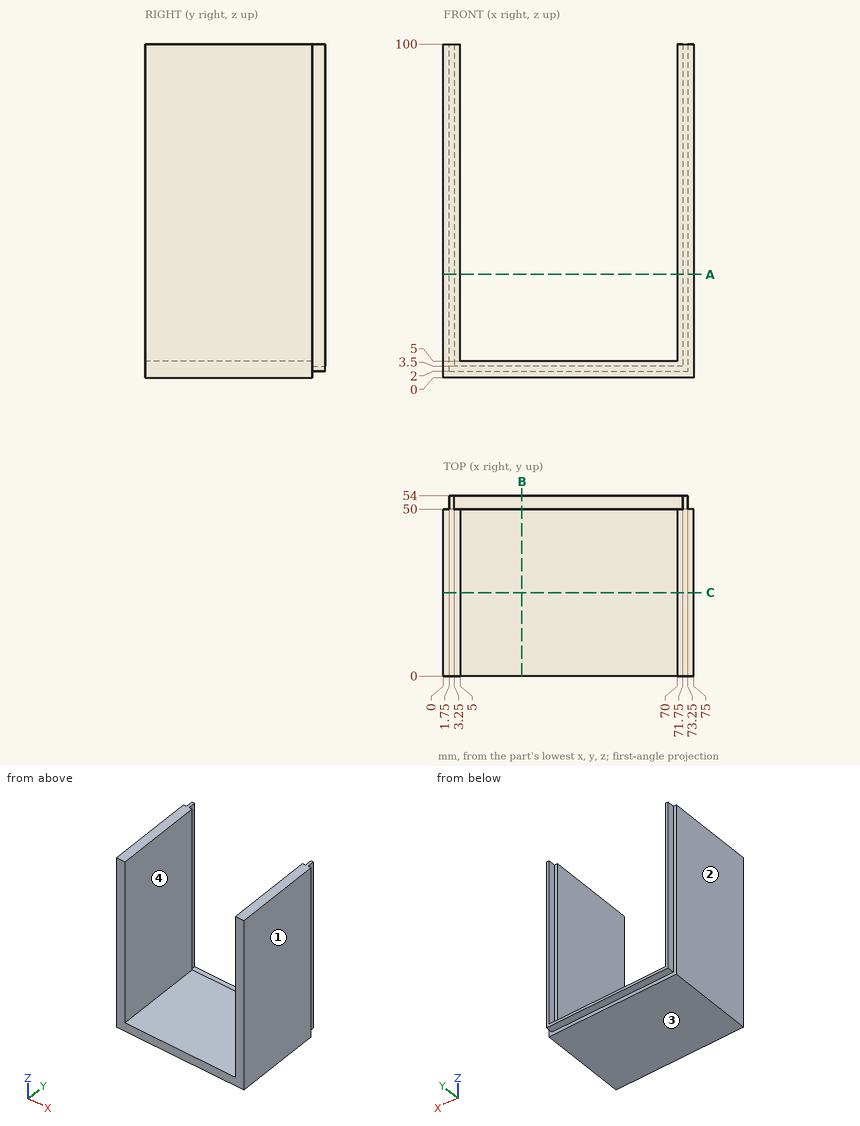
Study the drawing (mm; zero at the part's minimum x, y, z) and answer. Give positions to 0.01 mm unless a question says otherwise; leave off trailing zeros. Loops run counter-clockwise (first coordinate to the right, second up) from the corner with the lowest first, then second, coordinate; pieces in that order, holes last. Notation, with made-up numbers: M 67,88.5 L 82,88.5 A19 ccw 82,99.5 Z; hole C 45,33.5 d6. An arc over 180 degrees is marked long. Answer as CSV lines item,"result".
Item 1: The part is cut by section B-B (x = 23.5). Give the vertices of the cut face in (y, z).
Values follow:
outline,"M 0,0 L 50,0 L 50,2 L 54,2 L 54,3.5 L 50,3.5 L 50,5 L 0,5 Z"
Item 2: The part is cut by section A-A (z = 31). Give the vertices of the cut face in (x, y).
Values follow:
outline,"M 0,0 L 5,0 L 5,50 L 3.25,50 L 3.25,54 L 1.75,54 L 1.75,50 L 0,50 Z; M 70,0 L 75,0 L 75,50 L 73.25,50 L 73.25,54 L 71.75,54 L 71.75,50 L 70,50 Z"
Item 3: Straight lines are drawn through the part: line 1 along X through (y, z) = (51, 53); line 2 along X through (y, z) = (10, 15); line 3 along Z through (x, y) = (38, 17.5). For each, find the intervals that lie inside material, in ascending order. Write a range as [from, to].
Values follow:
line 1,"x = [1.75, 3.25], [71.75, 73.25]"
line 2,"x = [0, 5], [70, 75]"
line 3,"z = [0, 5]"
Item 4: The mould has two halves that part along X. Classify the marked faces 1, 2, 3 and 4: released by +X, released by -X, zero draft, split by the parting line, or undercut.
Values follow:
face 1,"released by +X"
face 2,"released by -X"
face 3,"zero draft"
face 4,"undercut"
Item 5: Given pin 1 Ø4.5 at (y, z) = (53, 66) entering from -X; pin 2 Ø2 at (x, y) = (56.5, 48) entering from +Z; pin 3 Ø3 at (y, z) = (52.5, 58.5) entering from +X, each flat-ended and moving along its own axis, determine where each tip first touches the part or whether it passes through.
Values follow:
pin 1,"stops at x = 1.75"
pin 2,"stops at z = 5"
pin 3,"stops at x = 73.25"
Item 6: The part is cut by section C-C (y = 25). Give the vertices of the cut face in (x, z), and give its area (4 significant figures).
Values follow:
outline,"M 0,0 L 75,0 L 75,100 L 70,100 L 70,5 L 5,5 L 5,100 L 0,100 Z"
area,"1,325 mm^2"
